The model under review builds one solid part; all positions refer to its coordinate system, in mm. Coordinates: 2 decimals unless noted, no trailing zeros. Return JSON: item names as keys, results as strings.
```python
from build123d import *
from OCP.BRepFilletAPI import BRepFilletAPI_MakeChamfer

# Parameters (mm, degrees)
CUT_EXTRUDE1_DEPTH = 28.440845468
CHAMFER1_SIZE      = 0.866025404
CHAMFER1_SIZE_2    = 1.5


with BuildPart() as part:
    # Sketch1 → Revolve1 (revolve)
    with BuildSketch(Plane(origin=(0, 0, 0), x_dir=(-1, 0, 0), z_dir=(0, 0, -1)), mode=Mode.PRIVATE) as revolve1_sk:
        Polygon((-8, -12.5), (0, -12.5), (0, 12.5), (-8, 12.5), (-8, 8.1), (-7.6, 8.1), (-7.6, 7), (-8, 7), (-8, -7), (-7.6, -7), (-7.6, -8.1), (-8, -8.1), align=None)
    revolve(revolve1_sk.sketch.rotate(Axis((0, -12.5, 0), (0, 1, 0)), 270), axis=Axis((0, -12.5, 0), (0, 1, 0)))

    # Sketch2 → Cut-Extrude1 (cut, through all)
    with BuildSketch(Plane.XZ.offset(12.5)):
        with BuildLine():
            Line((-1.690473047, 3.625231148), (-2.747018701, 5.891000616))
            ThreePointArc((-2.747018701, 5.891000616), (-3.25, 5.629165125), (-3.728246836, 5.324488288))
            Line((-3.728246836, 5.324488288), (-2.294305745, 3.276608177))
            ThreePointArc((-2.294305745, 3.276608177), (-2.828427125, 2.828427125), (-3.276608177, 2.294305745))
            Line((-3.276608177, 2.294305745), (-5.324488288, 3.728246836))
            ThreePointArc((-5.324488288, 3.728246836), (-5.629165125, 3.25), (-5.891000616, 2.747018701))
            Line((-5.891000616, 2.747018701), (-3.625231148, 1.690473047))
            ThreePointArc((-3.625231148, 1.690473047), (-3.863703305, 1.03527618), (-3.984778792, 0.348622971))
            Line((-3.984778792, 0.348622971), (-6.475265538, 0.566512328))
            ThreePointArc((-6.475265538, 0.566512328), (-6.5, 0), (-6.475265538, -0.566512328))
            Line((-6.475265538, -0.566512328), (-3.984778792, -0.348622971))
            ThreePointArc((-3.984778792, -0.348622971), (-3.863703305, -1.03527618), (-3.625231148, -1.690473047))
            Line((-3.625231148, -1.690473047), (-5.891000616, -2.747018701))
            ThreePointArc((-5.891000616, -2.747018701), (-5.629165125, -3.25), (-5.324488288, -3.728246836))
            Line((-5.324488288, -3.728246836), (-3.276608177, -2.294305745))
            ThreePointArc((-3.276608177, -2.294305745), (-2.828427125, -2.828427125), (-2.294305745, -3.276608177))
            Line((-2.294305745, -3.276608177), (-3.728246836, -5.324488288))
            ThreePointArc((-3.728246836, -5.324488288), (-3.25, -5.629165125), (-2.747018701, -5.891000616))
            Line((-2.747018701, -5.891000616), (-1.690473047, -3.625231148))
            ThreePointArc((-1.690473047, -3.625231148), (-1.03527618, -3.863703305), (-0.348622971, -3.984778792))
            Line((-0.348622971, -3.984778792), (-0.566512328, -6.475265538))
            ThreePointArc((-0.566512328, -6.475265538), (0, -6.5), (0.566512328, -6.475265538))
            Line((0.566512328, -6.475265538), (0.348622971, -3.984778792))
            ThreePointArc((0.348622971, -3.984778792), (1.03527618, -3.863703305), (1.690473047, -3.625231148))
            Line((1.690473047, -3.625231148), (2.747018701, -5.891000616))
            ThreePointArc((2.747018701, -5.891000616), (3.25, -5.629165125), (3.728246836, -5.324488288))
            Line((3.728246836, -5.324488288), (2.294305745, -3.276608177))
            ThreePointArc((2.294305745, -3.276608177), (2.828427125, -2.828427125), (3.276608177, -2.294305745))
            Line((3.276608177, -2.294305745), (5.324488288, -3.728246836))
            ThreePointArc((5.324488288, -3.728246836), (5.629165125, -3.25), (5.891000616, -2.747018701))
            Line((5.891000616, -2.747018701), (3.625231148, -1.690473047))
            ThreePointArc((3.625231148, -1.690473047), (3.863703305, -1.03527618), (3.984778792, -0.348622971))
            Line((3.984778792, -0.348622971), (6.475265538, -0.566512328))
            ThreePointArc((6.475265538, -0.566512328), (6.5, 0), (6.475265538, 0.566512328))
            Line((6.475265538, 0.566512328), (3.984778792, 0.348622971))
            ThreePointArc((3.984778792, 0.348622971), (3.863703305, 1.03527618), (3.625231148, 1.690473047))
            Line((3.625231148, 1.690473047), (5.891000616, 2.747018701))
            ThreePointArc((5.891000616, 2.747018701), (5.629165125, 3.25), (5.324488288, 3.728246836))
            Line((5.324488288, 3.728246836), (3.276608177, 2.294305745))
            ThreePointArc((3.276608177, 2.294305745), (2.828427125, 2.828427125), (2.294305745, 3.276608177))
            Line((2.294305745, 3.276608177), (3.728246836, 5.324488288))
            ThreePointArc((3.728246836, 5.324488288), (3.25, 5.629165125), (2.747018701, 5.891000616))
            Line((2.747018701, 5.891000616), (1.690473047, 3.625231148))
            ThreePointArc((1.690473047, 3.625231148), (1.03527618, 3.863703305), (0.348622971, 3.984778792))
            Line((0.348622971, 3.984778792), (0.566512328, 6.475265538))
            ThreePointArc((0.566512328, 6.475265538), (0, 6.5), (-0.566512328, 6.475265538))
            Line((-0.566512328, 6.475265538), (-0.348622971, 3.984778792))
            ThreePointArc((-0.348622971, 3.984778792), (-1.03527618, 3.863703305), (-1.690473047, 3.625231148))
        make_face()
    extrude(amount=-CUT_EXTRUDE1_DEPTH, mode=Mode.SUBTRACT)

    # Chamfer1
    chamfer1_edges_1 = [part.edges().sort_by_distance(p)[0] for p in [
        (0, 12.5, -8),
    ]]
    chamfer1_side_1 = [part.faces().sort_by_distance(p)[0] for p in [
        (0, 12.5, -7.982679492),
    ]]
    chamfer1_edges_2 = [part.edges().sort_by_distance(p)[0] for p in [
        (0, -12.5, -8),
    ]]
    chamfer1_side_2 = [part.faces().sort_by_distance(p)[0] for p in [
        (0, -12.5, -7.982679492),
    ]]
    chamfer1 = BRepFilletAPI_MakeChamfer(part.part.solid().wrapped)
    for e in chamfer1_edges_1:
        chamfer1.Add(CHAMFER1_SIZE - 0.0001, CHAMFER1_SIZE_2 - 0.0001, e.wrapped, chamfer1_side_1[0].wrapped)
    for e in chamfer1_edges_2:
        chamfer1.Add(CHAMFER1_SIZE_2 - 0.0001, CHAMFER1_SIZE - 0.0001, e.wrapped, chamfer1_side_2[0].wrapped)
    add(Compound.cast(chamfer1.Shape()), mode=Mode.REPLACE)  # a hair under: the kernel refuses the full size


solid = part.part
```
1. Insertion check: pin 1 Ø5 at (y, z) = (8.5, -6.5) entering from -X; pin 2 Ø2 at (x, y) = (2, -9) entering from +Z; pin 3 Ø1.5 at (y, z) = (4, -5) entering from -X. Each pin has a flat end and moves straight along its axis. Give the tip position at first contact, or say it passes through.
Check values:
{"pin 1": "x = -6.93", "pin 2": "z = 7.94", "pin 3": "x = -6.78"}
2. Add section C-C on x = 5. State how many separate pieces and enclosed holes the cut face has, plus the area to 3 significant figures.
Check values:
{"separate pieces": "4", "enclosed holes": "0", "area": "226 mm²"}
3. The part is to be moulded in two halves that separate along X. For faces 1 (the face through (-3, -12.5, -3)), 2 (the face through (-2.91, -7.56, 7.02)), 3 (the face through (-3.243, -0.175, 5.633)), say which applies: released by +X, released by -X, zero draft, split by the parting line, or undercut.
Check values:
{"face 1": "zero draft", "face 2": "split by the parting line", "face 3": "undercut"}
4. To check wall thickness, follow line 1 (X direction, y = -6.75, z = -0.25); line 2 (Z direction, x = -5, y = -5.25) (3 decimals); line 3 (X direction, y = -1, z = 5.5). State the ranges of each line that lie inside material, in increasing order.
Check values:
{"line 1": "-8 to -6.5, 6.5 to 8", "line 2": "-6.245 to -3.501, -2.332 to -0.437, 0.437 to 2.332, 3.501 to 6.245", "line 3": "-5.81 to -3.46, -2.56 to -0.48, 0.48 to 2.56, 3.46 to 5.81"}
